```python
from build123d import *

# Parameters (mm, degrees)
SKETCH1_R           = 10
BOSS_EXTRUDE1_DEPTH = 30
FILLET1_R           = 4
SKETCH2_W           = 60
SKETCH2_H           = 18
SKETCH2_W_2         = 57
SKETCH2_H_2         = 2.2
BOSS_EXTRUDE2_DEPTH = 40
SKETCH3_W           = 60
SKETCH3_H           = 18
BOSS_EXTRUDE3_DEPTH = 1
FILLET2_R           = 2
FILLET3_R           = 2


with BuildPart() as part:
    # Sketch1 → Boss-Extrude1 (new body)
    with BuildSketch(Plane(origin=(0, 0, 0), x_dir=(1, 0, 0), z_dir=(0, 1, 0))):
        with Locations(Location((0, 0, 0), (0, 0, 270))):
            Circle(SKETCH1_R)
    extrude(amount=BOSS_EXTRUDE1_DEPTH)

    # Fillet1
    fillet1_edges = [part.edges().sort_by_distance(p)[0] for p in [
        (0, 0, -10),
    ]]
    fillet(fillet1_edges, radius=FILLET1_R)

    # Sketch2 → Boss-Extrude2 (add)
    with BuildSketch(Plane(origin=(0, 30, 0), x_dir=(1, 0, 0), z_dir=(0, 1, 0))):
        Rectangle(SKETCH2_W, SKETCH2_H)
        with Locations((0, 1.9)):
            Rectangle(SKETCH2_W_2, SKETCH2_H_2, mode=Mode.SUBTRACT)
        with Locations((0, 5.9)):
            Rectangle(SKETCH2_W_2, SKETCH2_H_2, mode=Mode.SUBTRACT)
        with Locations((0, -2.1)):
            Rectangle(SKETCH2_W_2, SKETCH2_H_2, mode=Mode.SUBTRACT)
        with Locations((0, -6.1)):
            Rectangle(SKETCH2_W_2, SKETCH2_H_2, mode=Mode.SUBTRACT)
    extrude(amount=BOSS_EXTRUDE2_DEPTH)

    # Sketch3 → Boss-Extrude3 (add)
    with BuildSketch(Plane.XZ.offset(-30)):
        Rectangle(SKETCH3_W, SKETCH3_H)
    extrude(amount=BOSS_EXTRUDE3_DEPTH)

    # Fillet2
    fillet2_edges = [part.edges().sort_by_distance(p)[0] for p in [
        (-10, 29, 0),
        (10, 29, 0),
    ]]
    fillet(fillet2_edges, radius=FILLET2_R)

    # Fillet3
    # the kernel refuses this fillet: 2 mm, written as the material it adds along each edge
    with BuildSketch(Plane(origin=(-9.358898944, 30, 9), x_dir=(0, 0, 1), z_dir=(1, 0, 0))) as fillet3_piece_1_section:
        with BuildLine():
            CenterArc((FILLET3_R, -FILLET3_R), FILLET3_R, 90, 90)
            Line((0, -FILLET3_R), (0, 0))
            Line((0, 0), (FILLET3_R, 0))
        make_face()
    fillet3_piece_1 = extrude(amount=18.717797887, mode=Mode.PRIVATE)
    fillet3_piece_1 = fillet3_piece_1 & Plane(origin=(0, 30.566631584, 0), x_dir=(0, 0, 1), z_dir=(0, -1, 0)) * Cylinder(10, 46, mode=Mode.PRIVATE)
    add(fillet3_piece_1)
    with BuildSketch(Plane(origin=(9.358898944, 30, -9), x_dir=(0, 0, -1), z_dir=(-1, 0, 0))) as fillet3_piece_2_section:
        with BuildLine():
            CenterArc((FILLET3_R, -FILLET3_R), FILLET3_R, 90, 90)
            Line((0, -FILLET3_R), (0, 0))
            Line((0, 0), (FILLET3_R, 0))
        make_face()
    fillet3_piece_2 = extrude(amount=18.717797887, mode=Mode.PRIVATE)
    fillet3_piece_2 = fillet3_piece_2 & Plane(origin=(0, 30.566641093, 0), x_dir=(0, 0, 1), z_dir=(0, -1, 0)) * Cylinder(10, 46, mode=Mode.PRIVATE)
    add(fillet3_piece_2)


solid = part.part
```
Read the model definition and answer for the solid it produces. Units are mm, in the model's axes. A direction names the side the tool comes from. Coordinates: 2 decimals unless noted, no trailing zeros. Write each loop counter-clockwise with the first axis right and the second up, starting at its lowest first coordinate (ties: lowest second). Pieces come first, ordered by that corner, then holes. Notation, with made-up numbers: (-37, 34) - (3, 34) arc R19 cw to (3, 66) - close; hole circle Ø3 at (57, 4). An arc over 180 degrees is marked (long way). Answer as a JSON object with one key per item and string values. Group by question number.
1. A cutting plane is placed at C-C (x = -13). Determine the outline of the cut face in (y, z), plus the area to 3 significant figures.
2. The mould has two halves that part along Z. Classify faces 1 (the flat face through (0, 49, -9)), 2 (the flat face through (0, 30, -2)), 3 (the flat face through (30, 49, 0)): +Z half, -Z half, draft (parallel to the pull), parting line (faces both ways), or undercut.
3. Each of these flat-tipped pins is pushed along its axis until it touches: P1, Ø1.1, axis at x = 5.5, z = 6.5, coming from the +Y side; P2, Ø2, axis at y = 12.5, z = -5.5, coming from the +X side; P3, Ø12, axis at x = -9.5, y = 46, coming from the +Z side. Where does it stop, or does it pass through?
4. A cutting plane is placed at D-D (y = 24). Determine the outline of the cut face in (x, z), plus the area to 3 significant figures.
5. Which of the six approach directions +Z, -Z, +X, -X, +Y, -Y give full straight-line access (tool end or side, diameter ignored) to faces 4 (the flat face through (28.5, 50, 2)), 5 (the flat face through (0, 0, 0))?
6. A cutting plane is placed at A-A (y = 46). Determine the outline of the cut face in (x, z), plus the area to 3 significant figures.
7. A cutting plane is placed at B-B (z = 0). Determine the outline of the cut face in (x, y), plus the area to 3 significant figures.
8. Consider L1, parallel to Z at x = 19, y = 56.5; L2, parallel to X at y = 35.5, z = -1.5; L3, parallel to Y at x = 24, z = -3.75. Determine where each line is inside the solid, lowest interval first. Write a range as [from, to].
Worked out:
{
 "1": {"outline": "(29, -9) - (70, -9) - (70, -7) - (30, -7) - (30, -4.8) - (70, -4.8) - (70, -3) - (30, -3) - (30, -0.8) - (70, -0.8) - (70, 1) - (30, 1) - (30, 3.2) - (70, 3.2) - (70, 5) - (30, 5) - (30, 7.2) - (70, 7.2) - (70, 9) - (29, 9) - close", "area": "386 mm²"},
 "2": {"face 1": "-Z half", "face 2": "undercut", "face 3": "draft"},
 "3": {"P1": "stops at y = 30", "P2": "stops at x = 8.93", "P3": "stops at z = 9"},
 "4": {"outline": "circle Ø20 at (0, 0)", "area": "314 mm²"},
 "5": {"face 4": "+Y", "face 5": "+Z, -Z, +X, -X, -Y"},
 "6": {"outline": "(-30, -9) - (30, -9) - (30, 9) - (-30, 9) - close; hole (-28.5, -7) - (28.5, -7) - (28.5, -4.8) - (-28.5, -4.8) - close; hole (-28.5, -3) - (28.5, -3) - (28.5, -0.8) - (-28.5, -0.8) - close; hole (-28.5, 1) - (28.5, 1) - (28.5, 3.2) - (-28.5, 3.2) - close; hole (-28.5, 5) - (28.5, 5) - (28.5, 7.2) - (-28.5, 7.2) - close", "area": "578 mm²"},
 "7": {"outline": "(-30, 29) - (-12, 29) arc R2 cw to (-10, 27) - (-10, 4) arc R4 ccw to (-6, 0) - (6, 0) arc R4 ccw to (10, 4) - (10, 27) arc R2 cw to (12, 29) - (30, 29) - (30, 70) - (-30, 70) - close", "area": "3,030 mm²"},
 "8": {"L1": "z = [-9, -7], [-4.8, -3], [-0.8, 1], [3.2, 5], [7.2, 9]", "L2": "x = [-30, -28.5], [28.5, 30]", "L3": "y = [29, 70]"}
}
